CAD build for the part. Positions are in the model's coordinates, mm. A direction names the side the tool comes from. Round coordinates to 2 decimals unless told otherwise and drop trailing zeros. Loops run counter-clockwise (first coordinate to the right, second up) from the corner with the lowest first, then second, coordinate; pieces in that order, holes last. Notation, with made-up numbers: M 70.25,63 L 86.25,63 A29 ccw 86.25,84 Z; hole C 13.25,-12.75 d4. An arc over 180 degrees is marked long. Use a Markdown table: item, result. Add a question column.
(1) Band-saw the part on D-D, the plane z = 10.5. Write the cut outline in (x, y), and give its area (3 significant figures).
(2) Flat gauge pins, fed straight in: P1, Ø7, axis at y = 8.5, z = 11.5, coming from the +X side; P2, Ø4.5, axis at y = 9, z = 12, coming from the -X side; P3, Ø1, axis at y = 2, z = 10.5, coming from the -X side. Where does each tip first touch, or does it go through?
(3) Wall check: L1, parallel to Z at x = 33, y = -0.9; L2, parallel to X at y = 5.75, z = 19.25; L3, parallel to X at y = -1.75, z = 19. Give the ranges that are in metal, low to high.
(4) Two-plate mould, pull along X, no slides. Class faces 5 (the face through (14, 18, 15)), 6 (the face through (1, 20, 15)), 7 (the face through (-2, -4, 15)), 8 (the face through (36, -2, 15)): released by +X, released by -X, zero draft, split by the parting line, or undercut.
(5) Which spindle directions (+Z, -Z, +X, -X, +Y, -Y) get a long thin tool onto all of the face, cutting with end or side? Do faces 1 (the face through (23, 7, 15)), 2 (the face through (27, 10, 15)), 3 (the face through (13, 22, 15)), 4 (the face through (0, 10, 15)). Say none if no direction does.
(6) Band-saw the part on B-B, the plane z = 15.25. Write the cut outline in (x, y), and give its area (3 significant figures).
(7) Band-saw the part on A-A, the plane x = 33. Write the cut outline in (y, z).
(8) Band-saw the part on C-C, the plane y = 0.75. Write the cut outline in (x, z).
from build123d import *

# Parameters (mm, degrees)
BOSS_EXTRUDE1_DEPTH     = 23
CUT_EXTRUDE2_DEPTH      = 23
CUT_EXTRUDE2_DEPTH_BACK = 10
SKETCH4_W               = 3.5
SKETCH4_H               = 21
SKETCH5_W               = 45
SKETCH5_H               = 7.5
CUT_EXTRUDE3_DEPTH      = 26
SKETCH7_R               = 1.45
CUT_EXTRUDE4_DEPTH      = 26


with BuildPart() as part:
    # Sketch1 → Boss-Extrude1 (new body)
    with BuildSketch(Plane.XY):
        with BuildLine():
            Line((0, 3), (0, 17))
            ThreePointArc((0, 17), (1.464466094, 20.535533906), (5, 22))
            Line((5, 22), (22, 22))
            ThreePointArc((22, 22), (25.535533906, 20.535533906), (27, 17))
            Line((27, 17), (27, 3))
            ThreePointArc((27, 3), (27.878679656, 0.878679656), (30, 0))
            Line((30, 0), (36, 0))
            Line((36, 0), (36, -4))
            Line((36, -4), (23, -4))
            Line((23, -4), (23, 18))
            Line((23, 18), (4, 18))
            Line((4, 18), (4, -4))
            Line((4, -4), (-9, -4))
            Line((-9, -4), (-9, 0))
            Line((-9, 0), (-3, 0))
            ThreePointArc((-3, 0), (-0.878679656, 0.878679656), (0, 3))
        make_face()
    extrude(amount=BOSS_EXTRUDE1_DEPTH)

    # Sketch4 → Cut-Extrude2 (cut, two sides: drawn at the far end of the back side and taken through both)
    with BuildSketch(Plane.ZY.offset(-CUT_EXTRUDE2_DEPTH_BACK)):
        with Locations((5.75, 6.5)):
            Rectangle(SKETCH4_W, SKETCH4_H)
    extrude(amount=CUT_EXTRUDE2_DEPTH + CUT_EXTRUDE2_DEPTH_BACK, mode=Mode.SUBTRACT)

    # Sketch5 → Cut-Extrude3 (cut)
    with BuildSketch(Plane(origin=(0, 22, 0), x_dir=(1, 0, 0), z_dir=(0, 1, 0))):
        with Locations((13.5, -3.75)):
            Rectangle(SKETCH5_W, SKETCH5_H)
    extrude(amount=-CUT_EXTRUDE3_DEPTH, mode=Mode.SUBTRACT)

    # Sketch7 → Cut-Extrude4 (cut)
    with BuildSketch(Plane(origin=(0, 0, 0), x_dir=(1, 0, 0), z_dir=(0, 1, 0))):
        with Locations(Location((-6, -15.25, 0), (0, 0, 270))):
            Circle(SKETCH7_R)
        with Locations(Location((33, -15.25, 0), (0, 0, 180))):
            Circle(SKETCH7_R)
    extrude(amount=-CUT_EXTRUDE4_DEPTH, mode=Mode.SUBTRACT)


solid = part.part
Return value:
| question | item | result |
|---|---|---|
| 1 | outline | M -9,-4 L 4,-4 L 4,18 L 23,18 L 23,-4 L 36,-4 L 36,0 L 30,0 A3 cw 27,3 L 27,17 A5 ccw 22,22 L 5,22 A5 ccw 0,17 L 0,3 A3 cw -3,0 L -9,0 Z |
| 1 | area | 349 mm^2 |
| 2 | P1 | x = 27 |
| 2 | P2 | x = 0 |
| 2 | P3 | x = -0.4 |
| 3 | L1 | 7.5 to 13.8, 16.7 to 23 |
| 3 | L2 | 0 to 4, 23 to 27 |
| 3 | L3 | -9 to 4, 23 to 36 |
| 4 | face 5 | undercut |
| 4 | face 6 | released by -X |
| 4 | face 7 | zero draft |
| 4 | face 8 | released by +X |
| 5 | face 1 | +Z, -Z, -Y |
| 5 | face 2 | +Z, -Z, +X, +Y |
| 5 | face 3 | +Z, -Z, +X, -X, +Y |
| 5 | face 4 | +Z, -Z, -X, +Y |
| 6 | outline | M -9,-4 L -7.45,-4 L -7.45,0 L -9,0 Z; M -4.55,-4 L 4,-4 L 4,18 L 23,18 L 23,-4 L 31.55,-4 L 31.55,0 L 30,0 A3 cw 27,3 L 27,17 A5 ccw 22,22 L 5,22 A5 ccw 0,17 L 0,3 A3 cw -3,0 L -4.55,0 Z; M 34.45,-4 L 36,-4 L 36,0 L 34.45,0 Z |
| 6 | area | 326 mm^2 |
| 7 | outline | M -4,7.5 L 0,7.5 L 0,13.8 L -4,13.8 Z; M -4,16.7 L 0,16.7 L 0,23 L -4,23 Z |
| 8 | outline | M -1.02,7.5 L 4,7.5 L 4,23 L -1.02,23 Z; M 23,7.5 L 28.02,7.5 L 28.02,23 L 23,23 Z |
